For this review, take the finished solid that the model builds, in its own axes (mm). Face numbers are marked on the shaded views. Round coordinates to 2 decimals unless told otherwise and drop trailing zeros. Write each loop counter-clockwise with the first axis right and the second up, starting at its lowest first coordinate (ties: lowest second). Pieces come first, ordered by that corner, then holes. Notation, with made-up numbers: (13, 46) -> (22, 46) arc R21 ccw to (22, 81) -> close; hole circle Ø7 at (58.25, 49). An arc over 180 degrees is marked (long way). Answer in a Markdown table with one row per item. Add a question column.
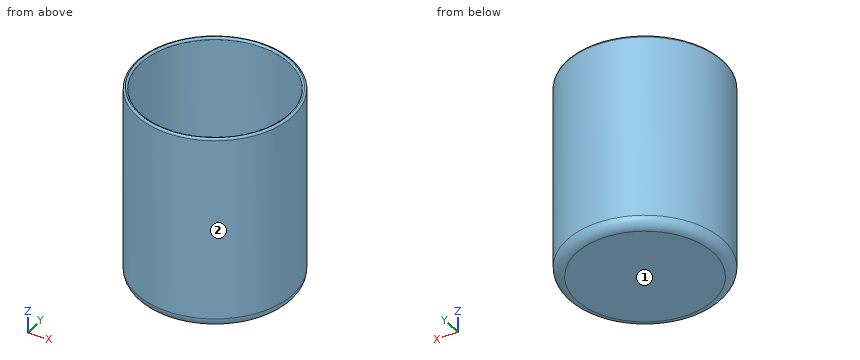
```python
from build123d import *

# Parameters (mm, degrees)
F0_R     = 40
F1_DEPTH = 100
F2_T     = -2
F3_R     = 1
F4_R     = 0.99999
F5_R     = 5


# Not quite as in the source:
# - a fillet or chamfer is up to 0.001 mm smaller than in the source, because OpenCascade refuses the exact size


with BuildPart() as f1:
    # F0 (on Top) → F1 (new body)
    with BuildSketch(Plane.XY):
        Circle(F0_R)
    extrude(amount=F1_DEPTH)

    # F2
    f2_openings = [f1.faces().sort_by_distance(p)[0] for p in [
        (0, 0, 100),
    ]]
    offset(amount=F2_T, openings=f2_openings)

    # F3
    f3_edges = [f1.edges().sort_by_distance(p)[0] for p in [
        (-38, 0, 100),
    ]]
    fillet(f3_edges, radius=F3_R)

    # F4 (radius 1 in the source; OpenCascade refuses exactly that, so slightly less here)
    f4_edges = [f1.edges().sort_by_distance(p)[0] for p in [
        (-40, 0, 100),
    ]]
    fillet(f4_edges, radius=F4_R)

    # F5
    f5_edges = [f1.edges().sort_by_distance(p)[0] for p in [
        (-40, 0, 0),
    ]]
    fillet(f5_edges, radius=F5_R)


solid = f1.part
```
1. We need section C-C (z = 87). Write out the cut boundary in (x, y), plus the area to 3 significant figures.
2. For L1, parallel to Y at x = 0, z = 79; L2, parallel to Z at x = -3, y = 8; L3, parallel to X at y = 6, z = 5, list the stretches that pass through material, from the lowest coordinate up. Write a range as [from, to].
3. Clearance check with flat-ended pins moving along their axes: pin 1 Ø4 at (x, z) = (-19.5, 34) entering from -Y; pin 2 Ø6 at (x, z) = (-1, 84) entering from +Y; pin 3 Ø4 at (x, z) = (2.5, 48.5) entering from -Y. State where each tip first meets the part, or that it passes through.
4. The part is to be moulded in two halves that separate along Z. For the marked faces 1 and 2, say which applies: pulls with the +Z half, pulls with the -Z half, needs draft (parallel to the pull), parting line crosses it, or undercut.
Response:
| question | item | result |
|---|---|---|
| 1 | outline | circle Ø80 at (0, 0); hole circle Ø76 at (0, 0) |
| 1 | area | 490 mm2 |
| 2 | L1 | [-40, -38], [38, 40] |
| 2 | L2 | [0, 2] |
| 2 | L3 | [-39.55, -37.52], [37.52, 39.55] |
| 3 | pin 1 | y = -35.97 |
| 3 | pin 2 | y = 40 |
| 3 | pin 3 | y = -40 |
| 4 | face 1 | pulls with the -Z half |
| 4 | face 2 | needs draft |
